from build123d import *

# Parameters (mm, degrees)
SKETCH_1_W               = 37.3
SKETCH_1_H               = 50.2
EXTRUDE_1_DEPTH          = 5
SKETCH_2_W               = 27.3
SKETCH_2_H               = 3.5
EXTRUDE_2_DEPTH          = 8.5
SKETCH_2_3_W             = 27.3
SKETCH_2_3_H             = 3.5
EXTRUDE_3_DEPTH          = 7.5
FILLET_1_R               = 1.2
FILLET_2_R               = 3
CUT_EXTRUDE_1_DEPTH      = 35.059983852
CUT_EXTRUDE_1_DEPTH_BACK = 35.059983852
SKETCH_4_R               = 1.6
SKETCH_5_W               = 4.5
SKETCH_5_H               = 4.5
CUT_EXTRUDE_2_DEPTH      = 1.5
SKETCH_6_R               = 1.45
CUT_EXTRUDE_3_DEPTH      = 35.059983852
CHAMFER_1_SIZE           = 1.5
CHAMFER_1_SIZE2          = 1.2
SKETCH_8_W               = 3
SKETCH_8_H               = 3
CUT_EXTRUDE_4_DEPTH      = 5
SKETCH_9_W               = 20.033877817
SKETCH_9_H               = 2
CUT_EXTRUDE_5_DEPTH      = 10


with BuildPart() as part:
    # 스케치1 → 보스-돌출1 (new body)
    with BuildSketch(Plane.XY):
        Rectangle(SKETCH_1_W, SKETCH_1_H)
    extrude(amount=EXTRUDE_1_DEPTH)

    # 스케치2 → 보스-돌출2 (add)
    with BuildSketch(Plane.XY):
        with Locations((0, -18.35)):
            Rectangle(SKETCH_2_W, SKETCH_2_H)
    extrude(amount=-EXTRUDE_2_DEPTH)

    # 스케치2<3> → 보스-돌출3 (add)
    with BuildSketch(Plane.XY):
        with Locations((0, 18.35)):
            Rectangle(SKETCH_2_3_W, SKETCH_2_3_H)
    extrude(amount=-EXTRUDE_3_DEPTH)

    # 필렛1
    fillet_1_edges = [part.edges().sort_by_distance(p)[0] for p in [
        (13.65, -20.1, -4.25),
        (-13.65, -20.1, -4.25),
        (-13.65, 20.1, -3.75),
        (13.65, 20.1, -3.75),
    ]]
    fillet(fillet_1_edges, radius=FILLET_1_R)

    # 필렛2
    fillet_2_edges = [part.edges().sort_by_distance(p)[0] for p in [
        (18.65, -25.1, 2.5),
        (-18.65, -25.1, 2.5),
        (-18.65, 25.1, 2.5),
        (18.65, 25.1, 2.5),
    ]]
    fillet(fillet_2_edges, radius=FILLET_2_R)

    # 스케치4 → 컷-돌출1 (cut, two sides: drawn at the far end of the back side and taken through both)
    with BuildSketch(Plane.XY.offset(5).offset(-CUT_EXTRUDE_1_DEPTH_BACK)):
        with Locations((8.15, 17.1)):
            Circle(SKETCH_4_R)
    extrude(amount=CUT_EXTRUDE_1_DEPTH + CUT_EXTRUDE_1_DEPTH_BACK, mode=Mode.SUBTRACT)

    # 스케치5 → 컷-돌출2 (cut)
    with BuildSketch(Plane(origin=(0, 0, -7.5), x_dir=(-1, 0, 0), z_dir=(0, 0, -1))):
        with Locations((-8.15, 17.1)):
            Rectangle(SKETCH_5_W, SKETCH_5_H)
    extrude(amount=-CUT_EXTRUDE_2_DEPTH, mode=Mode.SUBTRACT)

    # 스케치6 → 컷-돌출3 (cut, through all)
    with BuildSketch(Plane.XY.offset(5)):
        with Locations((-15.65, 22.1)):
            Circle(SKETCH_6_R)
        with Locations((15.65, 22.1)):
            Circle(SKETCH_6_R)
        with Locations((15.65, -22.1)):
            Circle(SKETCH_6_R)
        with Locations((-15.65, -22.1)):
            Circle(SKETCH_6_R)
    extrude(amount=-CUT_EXTRUDE_3_DEPTH, mode=Mode.SUBTRACT)

    # 모따기1
    chamfer_1_edges = [part.edges().sort_by_distance(p)[0] for p in [
        (-17.1, -22.1, 5),
        (14.2, -22.1, 5),
        (14.2, 22.1, 5),
        (-17.1, 22.1, 5),
    ]]
    chamfer_1_side = [part.faces().sort_by_distance(p)[0] for p in [
        (-0.035812285, -0.075139887, 5),
    ]]
    chamfer(chamfer_1_edges, length=CHAMFER_1_SIZE, length2=CHAMFER_1_SIZE2, reference=chamfer_1_side[0])

    # 스케치8 → 컷-돌출4 (cut)
    with BuildSketch(Plane.XY.offset(5)):
        with Locations((-11.15, 15.6)):
            Rectangle(SKETCH_8_W, SKETCH_8_H)
        with Locations((-11.15, -2.9)):
            Rectangle(SKETCH_8_W, SKETCH_8_H)
    extrude(amount=-CUT_EXTRUDE_4_DEPTH, mode=Mode.SUBTRACT)

    # 스케치9 → 컷-돌출5 (cut)
    with BuildSketch(Plane(origin=(0, 0, -7.5), x_dir=(-1, 0, 0), z_dir=(0, 0, -1))):
        with Locations((-10.016938909, 8.833508823)):
            Rectangle(SKETCH_9_W, SKETCH_9_H)
    extrude(amount=-CUT_EXTRUDE_5_DEPTH, mode=Mode.SUBTRACT)


solid = part.part
Geometry check sheet. Reference: the model listing, model coordinates, mm. A direction names the side the tool comes from. Round coordinates to 2 decimals unless told otherwise and drop trailing zeros. Loops run counter-clockwise (first coordinate to the right, second up) from the corner with the lowest first, then second, coordinate; pieces in that order, holes last.
Item 1: Access from +Z, -Z, +X, -X, +Y, -Y to the whole of each face (thin tool, end or side, straight path). Record for faces 5 (the flat face through (0, -16.6, -4)), 6 (the flat face through (8, 19, -6)), 7 (the flat face through (9, 9.834, 1)), 8 (the flat face through (-11, 17.1, 3)), 9 (the cylindrical face through (-13.289, 19.758, -3.802)).
Item 2: Cross-section at C-C on x = 4. Record the boundary of the cut face in (y, z), then the cut area to 3 significant figures.
Item 3: Mould release check, pull along X, two halves, no side actions. Record for faces 1 (the flat face through (10.4, 18, -7)), 2 (the cylindrical face through (7.942, 18.686, 0.645)), 3 (the cylindrical face through (-17.79, -24.2, 2.54)), 4 (the flat face through (9, 9, 2.5)): pulls with the +X half, pulls with the -X half, needs draft (parallel to the pull), parting line crosses it, or undercut.
Item 4: Gauge pin test, flat ends, axial feed: pin 1 (3 mm diameter, centred on x = -1, z = -5, fed in from -Y); pin 2 (2.5 mm diameter, centred on y = -18, z = -2.5, fed in from +X); pin 3 (10 mm diameter, centred on x = -7.5, y = 10.5, fed in from -Z). Record the tip position at first contact, or that the pin passes through.
Item 5: Cross-section at B-B on z = -4.5. Record the boundary of the cut face in (x, y), then the cut area to 3 significant figures.
Item 6: Cross-section at A-A on x = 8.15. Record the boundary of the cut face in (y, z), then the cut area to 3 significant figures.
Item 7: Thickness scan on line 1 (Y direction, x = -11.5, z = 4); line 2 (Y direction, x = -3, z = -6); line 3 (Y direction, x = 15.65, z = 1.15). Record the ranges inside material, lowest first.
Item 8: Cross-section at D-D on y = 1. Record the boundary of the cut face in (x, z).
Answer sheet:
1. face 5: -Z, +X, -X
1. face 6: -Z
1. face 7: -Z, +X
1. face 8: +Z
1. face 9: -Z, -X, +Y
2. outline: (-25.1, 0) - (-20.1, 0) - (-20.1, -8.5) - (-16.6, -8.5) - (-16.6, 0) - (7.83, 0) - (7.83, 2.5) - (9.83, 2.5) - (9.83, 0) - (16.6, 0) - (16.6, -7.5) - (20.1, -7.5) - (20.1, 0) - (25.1, 0) - (25.1, 5) - (-25.1, 5) - close
2. area: 302 mm2
3. face 1: undercut
3. face 2: undercut
3. face 3: pulls with the -X half
3. face 4: needs draft
4. pin 1: stops at y = -20.1
4. pin 2: stops at x = 13.65
4. pin 3: stops at z = 0
5. outline: (-13.65, -18.9) arc R1.2 ccw to (-12.45, -20.1) - (12.45, -20.1) arc R1.2 ccw to (13.65, -18.9) - (13.65, -16.6) - (-13.65, -16.6) - close; (-13.65, 16.6) - (6.63, 16.6) arc R1.6 cw (long way) to (9.67, 16.6) - (13.65, 16.6) - (13.65, 18.9) arc R1.2 ccw to (12.45, 20.1) - (-12.45, 20.1) arc R1.2 ccw to (-13.65, 18.9) - close
5. area: 184 mm2
6. outline: (-25.1, 0) - (-20.1, 0) - (-20.1, -8.5) - (-16.6, -8.5) - (-16.6, 0) - (7.83, 0) - (7.83, 2.5) - (9.83, 2.5) - (9.83, 0) - (15.5, 0) - (15.5, 5) - (-25.1, 5) - close; (18.7, -6) - (19.35, -6) - (19.35, -7.5) - (20.1, -7.5) - (20.1, 0) - (25.1, 0) - (25.1, 5) - (18.7, 5) - close
6. area: 269 mm2
7. line 1: y = -25.1 to -4.4, -1.4 to 14.1, 17.1 to 25.1
7. line 2: y = -20.1 to -16.6, 16.6 to 20.1
7. line 3: y = -25.1 to -23.55, -20.65 to 7.83, 9.83 to 20.65, 23.55 to 25.1
8. outline: (-18.65, 0) - (18.65, 0) - (18.65, 5) - (-18.65, 5) - close
